Autodesk Inventor part; units mm, degrees
ref_plane "YZ Plane" through (0, 0, 0) normal (1, 0, 0) x (0, 1, 0)
ref_plane "XZ Plane" through (0, 0, 0) normal (0, 1, 0) x (-1, 0, 0)
ref_plane "XY Plane" through (0, 0, 0) normal (0, 0, 1) x (1, 0, 0)
sketch "スケッチ1" plane through (0, 0, 0) normal (0, 1, 0) x (-1, 0, 0)
  arc A0 (0, -5) -> (-5, 0) centre (0, 0) ccw
  line L0 (0, -5) -> (-5, -5)
  line L1 (0, -5) -> (5, -5) construction
  line L2 (-5, -5) -> (-5, 0)
  dimension "d1" = 5
  dimension "d2" = 5
  dimension "d3" = 180
  dimension "d4" = 5
extrude "押し出し1" add sketch "スケッチ1" along normal blind 4.9
sketch "スケッチ2" plane through (0, 4.9, 0) normal (0, 1, 0) x (1, 0, 0)
  arc A0 (0, 5) -> (5, 0) centre (0, 0) ccw
  line L0 (0.0716, -4.9995) -> (0.0716, -6.9995)
  line L1 (0.0716, -6.9995) -> (3.5355, -3.5355)
  line L2 (0.0716, -6.9995) -> (4.9704, -6.9995) construction
  line L3 (0.0716, -4.9995) -> (3.5355, -3.5355)
  dimension "d7" = 2
  dimension "d8" = 45
extrude "押し出し2" add sketch "スケッチ2" against normal blind 4.9 contours A0 L1 L0
pattern_circular "円形状パターン1" count 3 over 100 about axis through (0, 0, 0) along (0, -1, 0) of "押し出し2"
sketch "スケッチ3" plane through (0, 4.9, 0) normal (0, 1, 0) x (1, 0, 0)
  point P0 (0, 0)
  point P1 (0, 0)
hole "穴1" at (0, 4.9, 0) direction (0, -1, 0) diameter 2 end through all
sketch "スケッチ4" plane through (5, 0, 0) normal (1, 0, 0) x (0, 0, -1)
  line L0 (0, 4.9) -> (5, 4.9)
  line L1 (5, 0) -> (5, 4.9)
  point P0 (0, 0)
  point P1 (2.5, 2.4)
  dimension "d28" = 2.5
  dimension "d29" = 2.5
hole "穴2" at (5, 2.4, -2.5) direction (-1, 0, 0) diameter 2.6 depth 5
sketch "スケッチ5" plane through (0, 4.9, 0) normal (0, 1, 0) x (1, 0, 0)
  point P0 (0, 0)
sketch "スケッチ7" plane through (0, 4.9, 0) normal (0, 1, 0) x (1, 0, 0)
  arc A0 (0, 5) -> (-4.936, 0.7977) centre (0, 0) ccw
  line L0 (0, 5) -> (-7, 5)
  line L1 (-7, 5) -> (-7, 4)
  line L2 (-7, 4) -> (-3, 4)
  line L3 (-3, 4) -> (0, 5)
  dimension "d35" = 7
  dimension "d36" = 1
extrude "押し出し4" add sketch "スケッチ7" against normal blind 4.9 contours A0 L2 L1 L0
equation "\"d9\" = atumi"
equation "\"d37\" = atumi"
properties part number "exp_latch_rod_rev0"
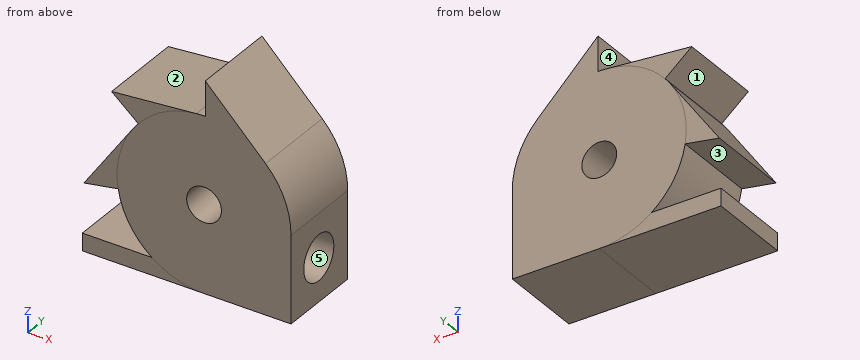
Geometry check sheet. Reference: the model listing, model coordinates, mm. Face numbers are marked on the shaded views. A direction names the side the tool comes from. Round coordinates to 2 decimals unless told otherwise and drop trailing zeros. Order: outer loops, then holes, each group sorted by start corner. A loop starts at its lowest first (then second) coordinate and runs counter-clockwise, first axis right, second up. Notation, with made-up numbers: (-3, -15.75) - (31, -15.75) arc R13 cw to (31, -6.75) - close; hole circle Ø1 at (-1.5, 74). An arc over 180 degrees is marked (long way). Use a Markdown table: item, result. Add a question column.
1) Section check D-D (z = -2.5). Record the cut outline in (x, y).
2) Set-up check for the marked faces 1, 2 and 3: record each of +Z, -Z, +X, -X, +Y, -Y from which the full face is reachable in a straight line by a thin tool's end or side.
3) Section check C-C (z = -0.25). Record the cut outline in (x, y), then the cut area to 3 significant figures.
4) Gauge pin test, flat ends, axial feed: P1, Ø2, axis at x = 1.5, y = 4.5, coming from the +Z side; P2, Ø1.3, axis at y = 3, z = -3, coming from the +X side; P3, Ø1.6, axis at x = 0, z = 0, coming from the -Y side; P4, Ø1.6, axis at y = 2.4, z = -2.5, coming from the -X side. Record the tip position at first contact, or that the pin passes through.
5) Section check A-A (y = 0.85). Record the cut outline in (x, z), then the cut area to 3 significant figures.
6) Mould release check, pull along Y, two halves, no side actions. Record for the marked faces 4 and 5: released by +Y, released by -Y, zero draft, split by the parting line, or undercut.
7) Thickness scan on line 1 along Y through (x, z) = (3.3, -2.5); line 2 along Z through (x, y) = (-4, 1.65); line 3 along Z through (x, y) = (-3.25, 3.05). Record the ranges inside material, lowest first.
8) Section check B-B (x = -5.5). Record the cut outline in (y, z).
Established:
| question | item | result |
|---|---|---|
| 1 | outline | (-4.33, 0) - (5, 0) - (5, 1.1) - (0, 1.1) - (0, 3.7) - (5, 3.7) - (5, 4.9) - (-4.33, 4.9) - close |
| 2 | face 1 | -X, +Y, -Y |
| 2 | face 2 | +Z, -X, +Y, -Y |
| 2 | face 3 | +Y, -Y |
| 3 | outline | (-6.28, 0) - (-0.97, 0) - (-0.97, 4.9) - (-6.28, 4.9) - close; (0.97, 0) - (5, 0) - (5, 4.9) - (0.97, 4.9) - close |
| 3 | area | 45.8 mm2 |
| 4 | P1 | z = 6.57 |
| 4 | P2 | x = 5 |
| 4 | P3 | through |
| 4 | P4 | x = -4.7 |
| 5 | outline | (-7, -5) - (5, -5) - (5, 0) arc R5 ccw to (3.54, 3.54) - (0.07, 7) - (0.07, 5) arc R5 ccw to (-0.44, 4.98) - (-5.32, 4.55) - (-3.78, 3.27) arc R5 ccw to (-4.1, 2.87) - (-6.91, -1.14) - (-4.94, -0.8) arc R5 ccw to (-3, -4) - (-7, -4) - close; hole circle Ø2 at (0, 0) |
| 5 | area | 93.3 mm2 |
| 6 | face 4 | zero draft |
| 6 | face 5 | undercut |
| 7 | line 1 | 0 to 1.1, 3.7 to 4.9 |
| 7 | line 2 | -5 to -4, -3 to 3, 3.45 to 4.67 |
| 7 | line 3 | -5 to -4, -3.8 to 4.73 |
| 8 | outline | (0, -5) - (4.9, -5) - (4.9, -4) - (0, -4) - close; (0, -0.9) - (4.9, -0.9) - (4.9, 0.86) - (0, 0.86) - close |
